Autodesk Inventor part; units mm, degrees
ref_plane "YZ Plane" through (0, 0, 0) normal (1, 0, 0) x (0, 1, 0)
ref_plane "XZ Plane" through (0, 0, 0) normal (0, 1, 0) x (-1, 0, 0)
ref_plane "XY Plane" through (0, 0, 0) normal (0, 0, 1) x (1, 0, 0)
sketch "스케치1" plane through (0, 0, 0) normal (0, 1, 0) x (-1, 0, 0)
  line L0 (-10, 10) -> (10, 10)
  line L1 (10, 10) -> (10, -10)
  line L2 (10, -10) -> (-10, -10)
  line L3 (-10, -10) -> (-10, 10)
  line L4 (-10, 10) -> (10, -10) construction
  line L5 (10, 10) -> (-10, -10) construction
  line L6 (-10, -10) -> (-15, -10)
  line L7 (-15, -10) -> (-15, 10)
  line L8 (-15, 10) -> (-10, 10)
  line L9 (-10, 10) -> (-10, -10)
  circle A0 centre (0, 0) radius 45.75
  dimension "d0" = 20
  dimension "d1" = 20
  dimension "d2" = 5
  dimension "d17" = 91.5
ref_plane "작업 평면2" through (-10, 20, -10) normal (-1, 0, 0) x (0, 0, 1)
sketch "스케치2" plane through (-10, 20, -10) normal (-1, 0, 0) x (0, 0, 1)
  line L0 (20, -100) -> (20, 0)
  line L1 (0, 0) -> (20, 0)
  line L2 (0, 0) -> (0, -100)
  line L3 (20, -100) -> (0, -100)
  circle A0 centre (10, -91) radius 4.5
  point P0 (10, -20)
  dimension "d7" = 9
  dimension "d8" = 9
ref_plane "작업 평면1" through (-10, 20, 10) normal (0, 0, 1) x (1, 0, 0)
sketch "스케치3" plane through (-10, 20, 10) normal (0, 0, 1) x (1, 0, 0)
  line L0 (20, -20) -> (25, -20)
  line L1 (25, -20) -> (25, 0)
  line L2 (0, 0) -> (25, 0)
  line L3 (0, -100) -> (0, 0)
  line L4 (20, -100) -> (0, -100)
  line L5 (20, -20) -> (20, -100)
  line L6 (25, -20) -> (25, 0)
  line L7 (25, 0) -> (0, 0)
  arc A0 (25, -20) -> (20, 0) centre (-10.6945, -18.2986) ccw
  line L8 (20, 0) -> (25, 0)
  line L9 (25, 0) -> (25, -20)
  point P0 (10, -20)
  point P1 (20, 0)
  point P2 (25, -16.5972)
extrude "돌출4" [suppressed]
extrude "돌출5" [suppressed]
extrude "돌출6" add sketch "스케치1" against normal blind 10
ref_plane "작업 평면3" through (10, 0, -10) normal (0, 0, 1) x (1, 0, 0)
sketch "스케치4" plane through (10, 0, -10) normal (0, 0, 1) x (1, 0, 0)
  line L0 (0, -5) -> (-10, -5)
  line L1 (-10, -5) -> (-10, -80)
  line L2 (0, -80) -> (-10, -80)
  line L3 (0, -5) -> (0, -80)
  line L4 (-10, 0) -> (0, 0)
  line L5 (0, 0) -> (5, 0)
  line L6 (5, 0) -> (5, 3.4028)
  arc A0 (5, 3.4028) -> (0, 20) centre (-30.6945, 1.7014) ccw
  line L7 (-10, 20) -> (0, 20)
  line L8 (-10, 20) -> (-10, 0)
  line L9 (0, -5) -> (5, -5)
  line L10 (5, -5) -> (5, 0)
  line L11 (5, 0) -> (0, 0)
  line L12 (0, 0) -> (0, -5)
  line L13 (-55.75, -5) -> (35.75, -5)
  line L14 (-10, 0) -> (-15, 0)
  line L15 (-15, 0) -> (-15, -5)
  line L16 (-15, -5) -> (-10, -5)
  line L17 (-10, -5) -> (-10, 0)
  line L18 (-15, 0) -> (-10, -5)
  line L19 (0, 0) -> (5, -5)
  dimension "d20" = 5
sketch "스케치5" plane through (0, 0, 0) normal (0, 1, 0) x (1, 0, 0)
  circle A0 centre (0, 0) radius 45.75
  line L0 (15, -10) -> (-10, -10)
  line L1 (-10, 10) -> (15, 10)
  line L2 (-12.2866, 10.5) -> (15, 10.5)
  line L3 (15, 10.5) -> (15, -10.5)
  line L4 (15, -10.5) -> (-12.2866, -10.5)
  line L5 (-12.2866, -10.5) -> (-12.2866, 10.5)
  line L6 (15, 10) -> (15, -10)
  line L7 (-10, -10) -> (-10, 10)
  dimension "d22" = 0.5
extrude "돌출7" [suppressed]
sketch "스케치6" plane through (-12.2866, 0, -10.5) normal (0, 0, 1) x (1, 0, 0)
  line L0 (7.2866, 0) -> (12.2866, -5)
  line L1 (7.2866, 0) -> (7.2866, -5)
  line L2 (7.2866, -5) -> (12.2866, -5)
  line L3 (22.2866, 0) -> (27.2866, -5)
  line L4 (22.2866, 0) -> (22.2866, -5)
  line L5 (22.2866, -5) -> (27.2866, -5)
  point P0 (12.2866, 0)
extrude "돌출8" [suppressed]
extrude "돌출9" add sketch "스케치4" along normal blind 20.5 and the other way blind 0.5 contours L19 L5 L10
ref_plane "작업 평면4" through (-12.2866, -5, -10.5) normal (0, 0, 1) x (1, 0, 0)
sketch "스케치7" plane through (-12.2866, -5, -10.5) normal (0, 0, 1) x (1, 0, 0)
  line L0 (7.2866, 0) -> (7.2866, 5)
  line L1 (0, 5) -> (7.2866, 5)
  line L2 (0, 5) -> (0, 0)
  line L3 (7.2866, 0) -> (0, 0)
  line L4 (0, 5) -> (7.2866, 5)
  line L5 (7.2866, 5) -> (7.2866, 0)
  line L6 (7.2866, 0) -> (0, 0)
  line L7 (0, 0) -> (0, 5)
  point P0 (12.2866, 5)
extrude "돌출10" add sketch "스케치7" along normal blind 21
sketch "스케치8" plane through (-5, 0, -10) normal (0, 0, 1) x (1, 0, 0)
  line L0 (0, 0) -> (0, -5)
  line L1 (20, -10) -> (-5, -10)
  line L2 (20, -5) -> (15, 0)
  line L3 (0, 0) -> (15, 0)
  line L4 (0, 0) -> (5, 0)
  line L5 (5, 0) -> (5, -10)
  line L6 (5, -10) -> (0, -10)
  line L7 (0, -10) -> (0, 0)
  line L8 (0, 0) -> (5, -10)
  line L9 (0, -5) -> (-5, -5)
  line L10 (-5, -5) -> (-5, -10)
  line L11 (20, -5) -> (20, -10)
  dimension "d33" = 5
extrude "돌출11" add sketch "스케치8" along normal blind 21
sketch "스케치9" plane through (0, 0, 0) normal (0, 1, 0) x (1, 0, 0)
  line L0 (10, -10) -> (-10, -10)
  line L1 (10, 10) -> (10, -10)
  line L2 (64.05, 10) -> (-64.05, 10)
  line L3 (-10, -64.05) -> (-10, 64.05)
  line L4 (-10, -10) -> (-10, 10)
  line L5 (-10, 10) -> (10, 10)
  line L6 (10, -10) -> (0, -10)
  line L7 (0, -10) -> (0, 10)
  line L8 (0, 10) -> (10, 10)
  line L9 (10, 10) -> (10, -10)
  point P0 (0, 0)
extrude "돌출12" cut sketch "스케치9" against normal blind 10 contours L0 L7 L2 L1
sketch "스케치10" plane through (10, 0, 10) normal (0, 0, -1) x (-1, 0, 0)
  line L0 (-5, 0) -> (0, 0)
  line L1 (0, 0) -> (0, -10)
  line L2 (-35.75, -10) -> (55.75, -10)
  line L3 (0, 0) -> (-5, 0)
  line L4 (-5, 0) -> (-5, -10)
  line L5 (-5, -10) -> (0, -10)
  line L6 (0, -10) -> (0, 0)
  line L7 (0, 0) -> (-5, -10)
  line L8 (10, 0) -> (15, 0)
  line L9 (15, 0) -> (15, -10)
  line L10 (15, -10) -> (10, -10)
  line L11 (10, -10) -> (10, 0)
  line L12 (15, 0) -> (10, -10)
  dimension "d38" = 5
extrude "돌출13" cut sketch "스케치10" along normal blind 20 contours L11 L8 L12
extrude "돌출14" cut sketch "스케치10" along normal blind 20 contours L1 L2 L7
sketch "스케치11" plane through (10, 0, 10) normal (0, 0, -1) x (-1, 0, 0)
  line L0 (-35.75, -10) -> (55.75, -10)
  line L1 (55.75, 0) -> (-35.75, 0)
  line L2 (0, 0) -> (0, -10)
  line L3 (10, -10) -> (10, 0)
  line L4 (0, 0) -> (10, 0)
  line L5 (10, 0) -> (10, -10)
  line L6 (10, -10) -> (0, -10)
  line L7 (0, -10) -> (0, 0)
  circle A0 centre (5, -5) radius 2.5
  dimension "d43" = 5
extrude "돌출15" add sketch "스케치11" along normal blind 20 contours A0
sketch "스케치12" plane through (0, 0, 0) normal (0, 0, 1) x (1, 0, 0)
  line L0 (-45.75, -10) -> (45.75, -10)
  line L1 (45.75, 0) -> (-45.75, 0)
  line L2 (-45.75, -10) -> (45.75, -10)
  line L3 (-45.75, 0) -> (45.75, 0)
  line L4 (45.75, 0) -> (45.75, -10)
  line L5 (45.75, -10) -> (-45.75, -10)
  line L6 (-45.75, -10) -> (-45.75, 0)
  point P0 (0, 0)
extrude "돌출16" cut sketch "스케치12" against normal blind 50
sketch "스케치13" plane through (0, 0, 0) normal (0, 0, -1) x (-1, 0, 0)
  line L0 (13.75, -2.95) -> (38.85, -2.95)
  line L1 (38.85, -2.95) -> (38.85, -7.05)
  line L2 (38.85, -7.05) -> (13.75, -7.05)
  line L3 (13.75, -7.05) -> (13.75, -2.95)
  line L4 (-41.1, -2.95) -> (-21, -2.95)
  line L5 (-21, -2.95) -> (-21, -7.05)
  line L6 (-21, -7.05) -> (-41.1, -7.05)
  line L7 (-41.1, -7.05) -> (-41.1, -2.95)
  line L8 (45.75, 0) -> (45.75, -10)
  line L9 (-45.75, 0) -> (-45.75, -10)
  line L10 (-45.75, 0) -> (-10, 0)
  line L11 (5, 0) -> (45.75, 0)
  point P0 (0, 0)
  dimension "d48" = 25.1
  dimension "d49" = 4.1
  dimension "d50" = 20.1
  dimension "d51" = 4.1
  dimension "d52" = 6.9
  dimension "d53" = 4.65
  dimension "d54" = 2.95
  dimension "d55" = 2.95
extrude "돌출17" cut sketch "스케치13" against normal blind 5
sketch "스케치14" plane through (0, 0, 0) normal (0, 0, -1) x (-1, 0, 0)
  line L0 (38.85, -2.95) -> (38.85, -7.05)
  line L1 (38.85, -7.05) -> (13.75, -7.05)
  line L2 (13.75, -7.05) -> (13.75, -2.95)
  line L3 (13.75, -2.95) -> (38.85, -2.95)
  line L4 (0, -10) -> (5, 0)
  line L5 (45.75, -10) -> (0, -10)
  line L6 (45.75, 0) -> (45.75, -10)
  line L7 (5, 0) -> (45.75, 0)
  line L8 (45.75, -2.95) -> (44.55, -2.95)
  line L9 (44.55, -2.95) -> (44.55, -7.05)
  line L10 (44.55, -7.05) -> (45.75, -7.05)
  line L11 (45.75, -7.05) -> (45.75, -2.95)
  line L12 (0, -12) -> (0, 2)
  point P0 (0, 0)
  dimension "d58" = 1.2
revolve "회전1" cut sketch "스케치14" angle 360 about axis through (0, -10, 0) along (0, 1, 0) contours L10 L9 L8 L6
sketch "스케치15" plane through (0, 0, 0) normal (0, 1, 0) x (1, 0, 0)
  circle A0 centre (-27.75, -16) radius 3.75
  circle A1 centre (-9.75, -16) radius 3.75
  circle A2 centre (9.25, -16) radius 3.75
  circle A3 centre (27.25, -16) radius 3.75
  circle A4 centre (-18.75, -29) radius 3.75
  circle A5 centre (0.25, -29) radius 3.75
  circle A6 centre (19.25, -29) radius 3.75
  line L0 (-44.55, 0) -> (-45.75, 0)
  line L1 (-45.75, 0) -> (-45.75, -49.8385)
  arc A7 (-45.75, 0) -> (45.75, 0) centre (0, 0) ccw
  line L2 (64.05, -10) -> (-64.05, -10)
  dimension "d60" = 7.5
  dimension "d61" = 7.5
  dimension "d62" = 7.5
  dimension "d63" = 7.5
  dimension "d64" = 7.5
  dimension "d65" = 7.5
  dimension "d66" = 7.5
  dimension "d67" = 18
  dimension "d68" = 18
  dimension "d69" = 19
  dimension "d70" = 18
  dimension "d71" = 9
  dimension "d72" = 19
  dimension "d73" = 19
  dimension "d74" = 13
  dimension "d75" = 13
  dimension "d76" = 13
  dimension "d77" = 6
  dimension "d78" = 6
sketch "스케치16" plane through (0, -10, 0) normal (0, -1, 0) x (1, 0, 0)
  circle A0 centre (27.25, 16) radius 3.75
  circle A1 centre (9.25, 16) radius 3.75
  circle A2 centre (-9.75, 16) radius 3.75
  circle A3 centre (-27.75, 16) radius 3.75
  circle A4 centre (-18.75, 29) radius 3.75
  circle A5 centre (0.25, 29) radius 3.75
  circle A6 centre (19.25, 29) radius 3.75
  point P0 (0, 0)
extrude "돌출19" cut sketch "스케치16" against normal blind 5
properties part number "new탄두윗판구멍1_2"
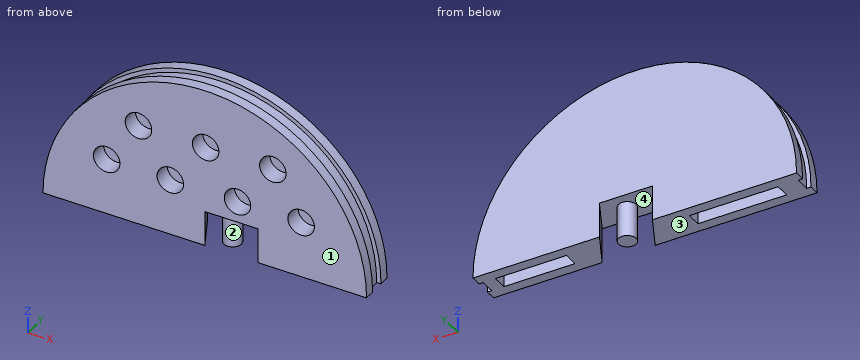
Could you check a few things on this model? Use its own coordinates, in mm. Face numbers are marked on the shaded views. A direction names the side the tool comes from. Give positions to 0.01 mm unless a question says otherwise; leave off trailing zeros. Order: outer loops, then holes, each group sorted by start corner. A loop starts at its lowest first (then second) coordinate and runs counter-clockwise, first axis right, second up.
1. We'd pull the mould along X, two halves only. Please class the marked faces 1 and 2: pulls with the +X half, pulls with the -X half, needs draft (parallel to the pull), parting line crosses it, or undercut.
2. Suppose I cut it at A-A (x = -11). List the corners of the cut face in (y, z) for me, plus the area to 3 significant figures.
3. For the marked faces 3 and 4, which set-ups out of +Z, -Z, +X, -X, +Y, -Y let a thin tool reach every point of the face, with its end or its side?
4. Suppose I cut it at C-C (x = -21). List the corners of the cut face in (y, z) for me.
5. Will these pins go through, and if not, where does the flat tip stop? P1, Ø3, axis at x = -32.5, y = -8, coming from the +Z side; P2, Ø7, axis at x = 9.25, z = 16, coming from the -Y side; P3, Ø2, axis at x = 33, y = -5, coming from the -Z side.
6. I need wall thicknesses on L1, parallel to Z at x = 0.25, y = -8.1; L2, parallel to X at y = -5.5, z = 2; L3, parallel to Z at x = -18.75, y = -6.9. Which ranges of each line are inside material? Lowest first, please.
7. Suppose I cut it at D-D (z = 29). List the corners of the cut face in (x, y) for me.
8. Suppose I cut it at B-B (z = 23.5). List the corners of the cut face in (x, y) for me.
Solved:
1. face 1: needs draft
1. face 2: undercut
2. outline: (-10, 0) - (0, 0) - (0, 44.41) - (-2.95, 44.41) - (-2.95, 43.17) - (-7.05, 43.17) - (-7.05, 44.41) - (-10, 44.41) - (-10, 19.54) - (-5, 19.54) - (-5, 12.46) - (-10, 12.46) - close
2. area: 404 mm2
3. face 3: -Z, +X, -X, +Y, -Y
3. face 4: -Z
4. outline: (-10, 0) - (-7.05, 0) - (-7.05, 5) - (-2.95, 5) - (-2.95, 0) - (0, 0) - (0, 40.65) - (-2.95, 40.65) - (-2.95, 39.29) - (-7.05, 39.29) - (-7.05, 40.65) - (-10, 40.65) - (-10, 32) - (-5, 32) - (-5, 26) - (-10, 26) - close
5. P1: stops at z = 33.65
5. P2: stops at y = -5
5. P3: stops at z = 5
6. L1: z = 10 to 25.25, 32.75 to 45.75
6. L2: x = -44.51 to -38.85, -13.75 to -2.25, 2.55 to 7.45, 12.75 to 21, 41.1 to 44.51
6. L3: z = 5 to 25.25, 32.75 to 40.41
7. outline: (-35.38, -10) - (-22.5, -10) - (-22.5, -5) - (-15, -5) - (-15, -10) - (-3.5, -10) - (-3.5, -5) - (4, -5) - (4, -10) - (15.5, -10) - (15.5, -5) - (23, -5) - (23, -10) - (35.38, -10) - (35.38, -7.05) - (33.82, -7.05) - (33.82, -2.95) - (35.38, -2.95) - (35.38, 0) - (-35.38, 0) - (-35.38, -2.95) - (-33.82, -2.95) - (-33.82, -7.05) - (-35.38, -7.05) - close
8. outline: (-39.25, -10) - (39.25, -10) - (39.25, -7.05) - (37.85, -7.05) - (37.85, -2.95) - (39.25, -2.95) - (39.25, 0) - (-39.25, 0) - (-39.25, -2.95) - (-37.85, -2.95) - (-37.85, -7.05) - (-39.25, -7.05) - close
